CAD build for the part. Positions are in the model's coordinates, mm. Face numbers are marked on the shaded views. A direction names the side the tool comes from. Give positions to 0.01 mm unless a question says otherwise; leave off trailing zeros. Write each loop counter-clockwise with the first axis right and the second up, starting at its lowest first coordinate (ties: lowest second). Pieces come first, ordered by that corner, then holes. Notation, with made-up numbers: (89, 0.5) -> (145, 0.5) arc R13 ccw to (145, 17.5) -> close; hole circle Ø4 at (-22.75, 87.5). An arc over 180 degrees is marked (long way). Answer in a Markdown table with one row per item. Add a question column.
```python
from build123d import *

# Parameters (mm, degrees)
PAD_DEPTH    = 12.5
SKETCH001_R  = 7.5
HOLE_DEPTH   = 25.001
PAD001_DEPTH = 97


with BuildPart() as part:
    # Sketch → Pad (new body, symmetric)
    with BuildSketch(Plane.XZ):
        with BuildLine():
            ThreePointArc((22.5, 0), (0, 22.5), (-22.5, 0))
            Line((-36.5, 0), (-22.5, 0))
            Line((-36.5, -18), (-36.5, 0))
            Line((-22.5, -32), (-36.5, -18))
            Line((22.5, -32), (-22.5, -32))
            Line((36.5, -18), (22.5, -32))
            Line((36.5, 0), (36.5, -18))
            Line((22.5, 0), (36.5, 0))
        make_face()
    extrude(amount=PAD_DEPTH, both=True)

    # Sketch001 (on Face10 of Pad) → Hole (cut, through all)
    with BuildSketch(Plane.XZ.offset(12.5)):
        Circle(SKETCH001_R)
    extrude(amount=-HOLE_DEPTH, mode=Mode.SUBTRACT)

    # Sketch002 (on Face5 of Pad) → Pad001 (join)
    with BuildSketch(Plane(origin=(0, 0, -32), x_dir=(1, 0, 0), z_dir=(0, 0, -1))):
        Polygon((-21, -2.872583), (-1.627417, 16.5), (1.627417, 16.5), (21, -2.872583), (21, -6.127417), (14.627417, -12.5), (-14.627417, -12.5), (-21, -6.127417), align=None)
    extrude(amount=PAD001_DEPTH)


solid = part.part
```
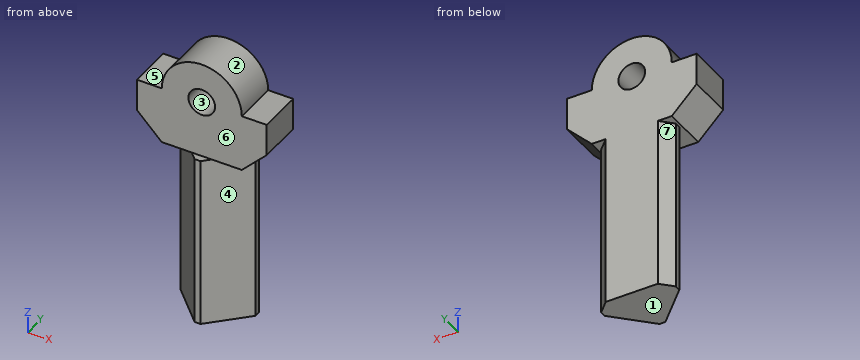
Item 1: Probe L1, parallel to Z at x = 0.5, y = -2; L2, parallel to X at y = 10.25, z = 0.5; L3, parallel to Z at x = -4, y = -7.5. List the from-to ranges inside material, lowest first. Write a range as from..to.
Item 2: Slice it at B-B, the plane z = -82. List the corners of the cut face in (x, y), then the cut area to 3 significant figures.
Item 3: Mould opens along Z. For the marked faces 1, 2 and 3 say: released by +Z, released by -Z, zero draft, split by the parting line, or undercut.
Item 4: Drop flat-ended pins along their axis: pin 1 Ø5 at (x, z) = (-22.5, -34) entering from -Y; pin 2 Ø15.5 at (x, y) = (-27.5, 0) entering from +Z; pin 3 Ø1 at (y, z) = (4.5, -58.5) entering from +X. Give the stop position or say it passes through.
Item 5: Which spindle directions (+Z, -Z, +X, -X, +Y, -Y) get a long thin tool onto all of the face, cutting with end or side? Do the marked faces 4, 5, 6 and 7. Say none if no direction does.
Item 6: Slice it at C-C, the plane y = -5.5. List the corners of the cut face in (x, z), then the cut area to 3 significant figures.
Item 7: Slice it at D-D, the plane x = 29. List the corners of the cut face in (y, z).
Item 8: Slice it at A-A, the plane x = 0. List the corners of the cut face in (y, z), then the cut area to 3 significant figures.
Answer key:
| question | item | result |
|---|---|---|
| 1 | L1 | z = -129..-7.48, 7.48..22.49 |
| 1 | L2 | x = -22.49..-7.48, 7.48..22.49 |
| 1 | L3 | z = -129..-6.34, 6.34..22.14 |
| 2 | outline | (-21, 2.87) -> (-1.63, -16.5) -> (1.63, -16.5) -> (21, 2.87) -> (21, 6.13) -> (14.63, 12.5) -> (-14.63, 12.5) -> (-21, 6.13) -> close |
| 2 | area | 802 mm² |
| 3 | face 1 | released by -Z |
| 3 | face 2 | released by +Z |
| 3 | face 3 | undercut |
| 4 | pin 1 | stops at y = -12.5 |
| 4 | pin 2 | stops at z = 10.78 |
| 4 | pin 3 | stops at x = 21 |
| 5 | face 4 | -Z, +X, -Y |
| 5 | face 5 | +Z, -X, +Y, -Y |
| 5 | face 6 | +Z, +X, -X, -Y |
| 5 | face 7 | -Z, -X, +Y |
| 6 | outline | (-36.5, -18) -> (-22.5, -32) -> (-12.63, -32) -> (-12.63, -129) -> (12.63, -129) -> (12.63, -32) -> (22.5, -32) -> (36.5, -18) -> (36.5, 0) -> (22.5, 0) arc R22.5 ccw to (-22.5, 0) -> (-36.5, 0) -> close; hole circle Ø15 at (0, 0) |
| 6 | area | 5,210 mm² |
| 7 | outline | (-12.5, -25.5) -> (12.5, -25.5) -> (12.5, 0) -> (-12.5, 0) -> close |
| 8 | outline | (-16.5, -129) -> (12.5, -129) -> (12.5, -7.5) -> (-12.5, -7.5) -> (-12.5, -32) -> (-16.5, -32) -> close; (-12.5, 7.5) -> (12.5, 7.5) -> (12.5, 22.5) -> (-12.5, 22.5) -> close |
| 8 | area | 3,800 mm² |
